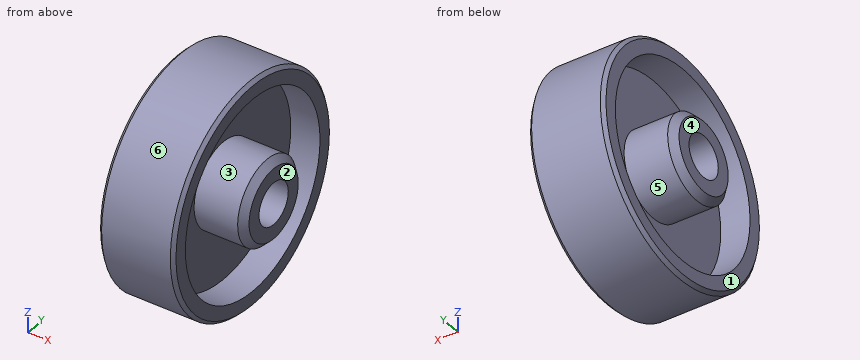
from build123d import *

# Parameters (mm, degrees)
F2_SIZE = 2.54
F3_SIZE = 5.08


with BuildPart() as f1:
    # F0 (on Front) → F1 (revolve)
    with BuildSketch(Plane.XZ):
        Polygon((28.575, 85.725), (-28.575, 85.725), (-28.575, 73.025), (-6.35, 73.025), (-6.35, 31.75), (-44.45, 31.75), (-44.45, 15.875), (44.45, 15.875), (44.45, 31.75), (6.35, 31.75), (6.35, 73.025), (28.575, 73.025), align=None)
    revolve(axis=Axis((-1.587497, 0, 0), (1, 0, 0)))

    # F2
    f2_edges = [f1.edges().sort_by_distance(p)[0] for p in [
        (-28.575, 0, -85.725),
        (28.575, 0, -85.725),
    ]]
    chamfer(f2_edges, length=F2_SIZE)

    # F3
    f3_edges = [f1.edges().sort_by_distance(p)[0] for p in [
        (44.45, 0, -31.75),
        (-44.45, 0, -31.75),
    ]]
    chamfer(f3_edges, length=F3_SIZE)


solid = f1.part
Geometry: final body of the model. Coordinates: model frame, mm. Face numbers are marked on the shaded views. A direction names the side the tool comes from. Give positions to 0.01 mm unless a question says otherwise; leave off trailing zeros. Loops run counter-clockwise (first coordinate to the right, second up) from the corner with the lowest first, then second, coordinate; pieces in that order, holes last. Notation, with made-up numbers: (73, 66.25) -> (94, 66.25) arc R21 cw to (94, 80.25) -> close; hole circle Ø10 at (56, -11.5). An arc over 180 degrees is marked (long way). Put each result on its own line as item: value.
1. Ray query, line 1 along Z through (x, y) = (14.5, 0) (3 decimals); line 2 along Y through (x, z) = (17.5, -22); line 3 along X through (y, z) = (-33, 63). Return the intervals inside material, ascending. Write a range as [from, to].
Taken from the geometry:
line 1: z = [-85.725, -73.025], [-31.75, -15.875], [15.875, 31.75], [73.025, 85.725]
line 2: y = [-82.85, -69.63], [-22.89, 22.89], [69.63, 82.85]
line 3: x = [-6.35, 6.35]
2. Pull-direction query (Y, two-part tool) for the marked faces 4, 5 and 6; classes: released by +Y, released by -Y, zero draft, split by the parting line, or undercut.
Taken from the geometry:
face 4: zero draft
face 5: undercut
face 6: split by the parting line
3. Cut plane C-C (x = -37). Return the cut outline in (y, z) (3 decimals), plus the area to 3 significant figures.
Taken from the geometry:
outline: circle Ø63.5 at (0, 0); hole circle Ø31.75 at (0, 0)
area: 2,380 mm2
4. Set-up query: the marked faces 1, 2 and 3. Return all of +Z, -Z, +X, -X, +Y, -Y with unobstructed straight access to the full face (end or side cutting, diameter ignored); none if empty.
Taken from the geometry:
face 1: -X
face 2: +Z, -Z, +X, +Y, -Y
face 3: +X
5. Pin query (flat end, axial travel): P1, Ø3, axis at x = -20, z = -30.5, coming from the +Y side; P2, Ø1, axis at x = 18, y = 56, coming from the +Z side; P3, Ø1.5, axis at y = -58.5, z = -37.5, coming from the -X side. Return the tip coordinate at first contact, or that it passes through.
Taken from the geometry:
P1: stops at y = 80.67
P2: stops at z = 65.33
P3: stops at x = -6.35
